Source: CAD feature listing. Evaluate the final solid. Frame: model axes, mm. Give positions to 0.01 mm unless a question says otherwise; leave off trailing zeros. Write each loop counter-clockwise with the first axis right and the second up, starting at its lowest first coordinate (ties: lowest second). Pieces come first, ordered by that corner, then holes. Notation, with made-up numbers: M 62,86.5 L 77,86.5 A23 cw 77,108.5 Z; hole C 27.25,0.25 d2. An arc over 180 degrees is marked long. Return JSON: item names as keys, results as strings.
```python
from build123d import *

# Parameters (mm, degrees)
SKETCH1_W               = 65
SKETCH1_H               = 65
BOSS_EXTRUDE1_DEPTH     = 1.5
SKETCH2_R               = 2.5
CUT_EXTRUDE1_DEPTH      = 2.5
CUT_EXTRUDE1_DEPTH_BACK = 2.5
CUT_EXTRUDE2_DEPTH      = 2.5
CUT_EXTRUDE2_DEPTH_BACK = 2.5
SKETCH4_R               = 3.5
CUT_EXTRUDE3_DEPTH      = 2.5
CUT_EXTRUDE3_DEPTH_BACK = 2.5
CUT_EXTRUDE4_DEPTH      = 2.5
CUT_EXTRUDE4_DEPTH_BACK = 2.5
FILLET1_R               = 2


with BuildPart() as part:
    # Sketch1 → Boss-Extrude1 (new body, symmetric)
    with BuildSketch(Plane(origin=(0, 0, 0), x_dir=(1, 0, 0), z_dir=(0, 1, 0))):
        Rectangle(SKETCH1_W, SKETCH1_H)
    extrude(amount=BOSS_EXTRUDE1_DEPTH, both=True)

    # Sketch2 → Cut-Extrude1 (cut, two sides)
    with BuildSketch(Plane(origin=(0, 0, 0), x_dir=(1, 0, 0), z_dir=(0, 1, 0))) as cut_extrude1_sk:
        Circle(SKETCH2_R)
        with Locations((0, 10)):
            Circle(SKETCH2_R)
        with Locations((0, -10)):
            Circle(SKETCH2_R)
        with Locations((0, -20)):
            Circle(SKETCH2_R)
        with Locations((-10, 0)):
            Circle(SKETCH2_R)
        with Locations((-10, 20)):
            Circle(SKETCH2_R)
        with Locations((-10, -20)):
            Circle(SKETCH2_R)
        with Locations((-20, 20)):
            Circle(SKETCH2_R)
        with Locations((-20, -20)):
            Circle(SKETCH2_R)
        with Locations((10, 0)):
            Circle(SKETCH2_R)
        with Locations((10, 20)):
            Circle(SKETCH2_R)
        with Locations((10, -20)):
            Circle(SKETCH2_R)
        with Locations((20, 20)):
            Circle(SKETCH2_R)
        with Locations((20, -20)):
            Circle(SKETCH2_R)
    extrude(amount=CUT_EXTRUDE1_DEPTH, mode=Mode.SUBTRACT)
    extrude(cut_extrude1_sk.sketch, amount=-CUT_EXTRUDE1_DEPTH_BACK, mode=Mode.SUBTRACT)

    # Sketch3 → Cut-Extrude2 (cut, two sides)
    with BuildSketch(Plane(origin=(0, 0, 0), x_dir=(1, 0, 0), z_dir=(0, 1, 0))) as cut_extrude2_sk:
        with BuildLine():
            Line((22.5, 10), (22.5, -10))
            ThreePointArc((22.5, -10), (20, -12.5), (17.5, -10))
            Line((17.5, -10), (17.5, 10))
            ThreePointArc((17.5, 10), (20, 12.5), (22.5, 10))
        make_face()
        with BuildLine():
            Line((-22.5, 10), (-22.5, -10))
            ThreePointArc((-22.5, -10), (-20, -12.5), (-17.5, -10))
            Line((-17.5, -10), (-17.5, 10))
            ThreePointArc((-17.5, 10), (-20, 12.5), (-22.5, 10))
        make_face()
    extrude(amount=CUT_EXTRUDE2_DEPTH, mode=Mode.SUBTRACT)
    extrude(cut_extrude2_sk.sketch, amount=-CUT_EXTRUDE2_DEPTH_BACK, mode=Mode.SUBTRACT)

    # Sketch4 → Cut-Extrude3 (cut, two sides)
    with BuildSketch(Plane(origin=(0, 0, 0), x_dir=(1, 0, 0), z_dir=(0, 1, 0))) as cut_extrude3_sk:
        with Locations((0, 20)):
            Circle(SKETCH4_R)
    extrude(amount=CUT_EXTRUDE3_DEPTH, mode=Mode.SUBTRACT)
    extrude(cut_extrude3_sk.sketch, amount=-CUT_EXTRUDE3_DEPTH_BACK, mode=Mode.SUBTRACT)

    # Sketch5 → Cut-Extrude4 (cut, two sides)
    with BuildSketch(Plane(origin=(0, 0, 0), x_dir=(1, 0, 0), z_dir=(0, 1, 0))) as cut_extrude4_sk:
        with BuildLine():
            ThreePointArc((-26, -23), (-27.5, -24.5), (-29, -23))
            Line((-29, -23), (-29, -17))
            ThreePointArc((-29, -17), (-27.5, -15.5), (-26, -17))
            Line((-26, -17), (-26, -23))
        make_face()
        with BuildLine():
            Line((26, 3), (26, -3))
            ThreePointArc((26, -3), (27.5, -4.5), (29, -3))
            Line((29, -3), (29, 3))
            ThreePointArc((29, 3), (27.5, 4.5), (26, 3))
        make_face()
        with BuildLine():
            Line((26, 23), (26, 17))
            ThreePointArc((26, 17), (27.5, 15.5), (29, 17))
            Line((29, 17), (29, 23))
            ThreePointArc((29, 23), (27.5, 24.5), (26, 23))
        make_face()
        with BuildLine():
            Line((-26, 23), (-26, 17))
            ThreePointArc((-26, 17), (-27.5, 15.5), (-29, 17))
            Line((-29, 17), (-29, 23))
            ThreePointArc((-29, 23), (-27.5, 24.5), (-26, 23))
        make_face()
        with BuildLine():
            Line((-26, 3), (-26, -3))
            ThreePointArc((-26, -3), (-27.5, -4.5), (-29, -3))
            Line((-29, -3), (-29, 3))
            ThreePointArc((-29, 3), (-27.5, 4.5), (-26, 3))
        make_face()
        with BuildLine():
            Line((29, -17), (29, -23))
            ThreePointArc((29, -23), (27.5, -24.5), (26, -23))
            Line((26, -23), (26, -17))
            ThreePointArc((26, -17), (27.5, -15.5), (29, -17))
        make_face()
    extrude(amount=CUT_EXTRUDE4_DEPTH, mode=Mode.SUBTRACT)
    extrude(cut_extrude4_sk.sketch, amount=-CUT_EXTRUDE4_DEPTH_BACK, mode=Mode.SUBTRACT)

    # Fillet1
    fillet1_edges = [part.edges().sort_by_distance(p)[0] for p in [
        (32.5, 0, 32.5),
        (-32.5, 0, 32.5),
        (-32.5, 0, -32.5),
        (32.5, 0, -32.5),
    ]]
    fillet(fillet1_edges, radius=FILLET1_R)


solid = part.part
```
1) Line query: line 1 (X direction, y = -0.15, z = 3); line 2 (Z direction, x = -10, y = -0.4); line 3 (Z direction, x = -10.5, y = 0.25). Output: solid intervals per line, ascending. Write a range as [from, to].
Numbers:
{"line 1": "x = [-32.5, -29], [-26, -22.5], [-17.5, 17.5], [22.5, 26], [29, 32.5]", "line 2": "z = [-32.5, -22.5], [-17.5, -2.5], [2.5, 17.5], [22.5, 32.5]", "line 3": "z = [-32.5, -22.45], [-17.55, -2.45], [2.45, 17.55], [22.45, 32.5]"}
2) Cut plane C-C, the plane z = 20. Give the number of separate pieces and of enclosed holes in the cut face, then the cut area to 3 significant figures.
Numbers:
{"separate pieces": "8", "enclosed holes": "0", "area": "102 mm²"}
3) Cut plane D-D, the plane x = 27.5. Return the cut outline in (y, z).
Numbers:
{"outline": "M -1.5,-32.5 L 1.5,-32.5 L 1.5,-24.5 L -1.5,-24.5 Z; M -1.5,-15.5 L 1.5,-15.5 L 1.5,-4.5 L -1.5,-4.5 Z; M -1.5,4.5 L 1.5,4.5 L 1.5,15.5 L -1.5,15.5 Z; M -1.5,24.5 L 1.5,24.5 L 1.5,32.5 L -1.5,32.5 Z"}
4) Cut plane B-B, the plane z = 5.5. Return the cut outline in (x, y), then the cut area to 3 significant figures.
Numbers:
{"outline": "M -32.5,-1.5 L -22.5,-1.5 L -22.5,1.5 L -32.5,1.5 Z; M -17.5,-1.5 L 17.5,-1.5 L 17.5,1.5 L -17.5,1.5 Z; M 22.5,-1.5 L 32.5,-1.5 L 32.5,1.5 L 22.5,1.5 Z", "area": "165 mm²"}
5) Cut plane A-A, the plane x = -10. Return the cut outline in (y, z).
Numbers:
{"outline": "M -1.5,-32.5 L 1.5,-32.5 L 1.5,-22.5 L -1.5,-22.5 Z; M -1.5,-17.5 L 1.5,-17.5 L 1.5,-2.5 L -1.5,-2.5 Z; M -1.5,2.5 L 1.5,2.5 L 1.5,17.5 L -1.5,17.5 Z; M -1.5,22.5 L 1.5,22.5 L 1.5,32.5 L -1.5,32.5 Z"}
